Model file for the job. Use its own axes, mm. Face numbers are marked on the shaded views. Give positions to 0.01 mm unless a question says otherwise; leave off trailing zeros. Loops run counter-clockwise (first coordinate to the right, second up) from the corner with the lowest first, then second, coordinate; pieces in that order, holes last. Notation, with made-up numbers: (52.5, 34.25) -> (81.5, 34.25) arc R13 cw to (81.5, 50.25) -> close; hole circle Ø7 at (57.5, 77). An arc over 180 degrees is marked (long way). Use CSV: the item, a comma, the result in double quotes. Start each with the question number.
(1) Flat gauge pins, fed straight in: pin 1 (4.5 mm diameter, centred on y = -69.5, z = -6, fed in from -X); pin 2 (6 mm diameter, centred on x = 3.5, z = 4, fed in from +Y); pin 3 (3 mm diameter, centred on y = -69.5, z = -8.5, fed in from +X). Where does each tip first touch, or does it go through?
(2) Cut at A-A on y = 8. Write the cut outline in (x, z), then the cut area to 3 significant figures.
(3) Cut at B-B on z = -11.75. Write the cut outline in (x, y), then the cut area to 3 significant figures.
(4) Pull direction X, two halves, no side cores. Call the marked faces 1, 2, 3 and 4: pulls with the +X half, pulls with the -X half, needs draft (parallel to the pull), parting line crosses it, or undercut.
(5) Cut at C-C on x = 15. Write the cut outline in (y, z), then the cut area to 3 significant figures.
(6) Drill centre lines: probe 1 along Y at (x, z) = (1.5, -4.75); probe 2 along Y at (x, z) = (0, 8); probe 3 along Z at (x, y) = (-31, 64). Where is each one in solid material? Low to high.
(7) Cut at D-D on x = -64.5. Write the cut outline in (y, z), then the cut area to 3 significant figures.
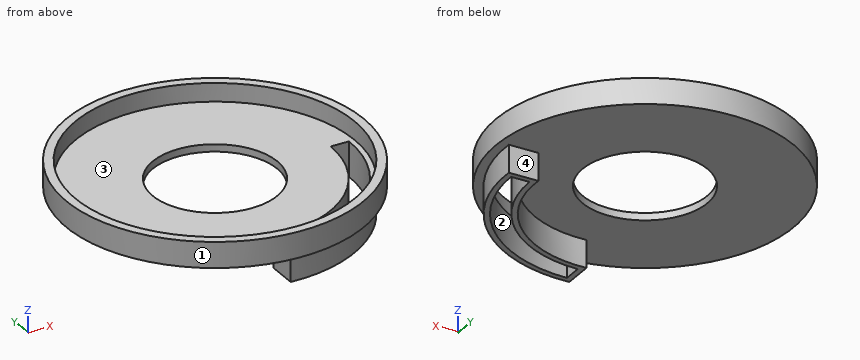
from build123d import *

# Parameters (mm, degrees)
SKETCH_1_R           = 76.1
SKETCH_1_R_2         = 34
EXTRUDE_1_DEPTH      = 4
EXTRUDE_2_DEPTH      = 10
EXTRUDE_2_DEPTH_BACK = 4
SKETCH_2_R           = 81.1
SKETCH_2_R_2         = 76.1
CUT_EXTRUDE_1_DEPTH  = 5
EXTRUDE_3_DEPTH      = 15


with BuildPart() as part:
    # 스케치1 → 보스-돌출1 (new body)
    with BuildSketch(Plane.XY):
        Circle(SKETCH_1_R)
        Circle(SKETCH_1_R_2, mode=Mode.SUBTRACT)
    extrude(amount=EXTRUDE_1_DEPTH)

    # 스케치2 → 보스-돌출2 (add, two sides: drawn at the far end of the back side and taken through both)
    with BuildSketch(Plane.XY.offset(4).offset(-EXTRUDE_2_DEPTH_BACK)):
        Circle(SKETCH_2_R)
        Circle(SKETCH_2_R_2, mode=Mode.SUBTRACT)
    extrude(amount=EXTRUDE_2_DEPTH + EXTRUDE_2_DEPTH_BACK)

    # 스케치3 → 컷-돌출1 (cut)
    with BuildSketch(Plane.XY.offset(4)):
        with BuildLine():
            Line((63, 0), (73.1, 0))
            ThreePointArc((73.1, 0), (51.689505705, -51.689505705), (0, -73.1))
            Line((0, -73.1), (0, -63))
            ThreePointArc((0, -63), (44.547727215, -44.547727215), (63, 0))
        make_face()
    extrude(amount=-CUT_EXTRUDE_1_DEPTH, mode=Mode.SUBTRACT)

    # 스케치4 → 보스-돌출3 (add)
    with BuildSketch(Plane(origin=(0, 0, 0), x_dir=(-1, 0, 0), z_dir=(0, 0, -1))):
        with BuildLine():
            Line((-59.924953066, 3), (-76.040844288, 3))
            ThreePointArc((-76.040844288, 3), (-53.810826048, -53.810826048), (3, -76.040844288))
            Line((3, -76.040844288), (3, -59.924953066))
            ThreePointArc((3, -59.924953066), (-42.426406871, -42.426406871), (-59.924953066, 3))
        make_face()
        with BuildLine():
            Line((-63, 0), (-73.1, 0))
            ThreePointArc((-73.1, 0), (-51.689505705, -51.689505705), (0, -73.1))
            Line((0, -73.1), (0, -63))
            ThreePointArc((0, -63), (-44.547727215, -44.547727215), (-63, 0))
        make_face(mode=Mode.SUBTRACT)
    extrude(amount=EXTRUDE_3_DEPTH)


solid = part.part
Check result:
1,pin 1,"x = -3"
1,pin 2,"y = 81.1"
1,pin 3,"x = 34.16"
2,outline,"(-80.7, 0) -> (-33.05, 0) -> (-33.05, 4) -> (-75.68, 4) -> (-75.68, 14) -> (-80.7, 14) -> close; (33.05, 0) -> (80.7, 0) -> (80.7, 14) -> (75.68, 14) -> (75.68, 4) -> (33.05, 4) -> close"
2,area,"482 mm²"
3,outline,"(-3, -76.04) arc R76.1 ccw to (76.04, 3) -> (59.92, 3) arc R60 cw to (-3, -59.92) -> close; hole (0, -73.1) arc R73.1 ccw to (73.1, 0) -> (63, 0) arc R63 cw to (0, -63) -> close"
3,area,"738 mm²"
4,face 1,"parting line crosses it"
4,face 2,"undercut"
4,face 3,"undercut"
4,face 4,"needs draft"
5,outline,"(-79.7, 0) -> (-74.61, 0) -> (-74.61, -15) -> (-71.54, -15) -> (-71.54, 4) -> (-74.61, 4) -> (-74.61, 14) -> (-79.7, 14) -> close; (-61.19, -15) -> (-58.09, -15) -> (-58.09, 0) -> (-30.51, 0) -> (-30.51, 4) -> (-61.19, 4) -> close; (30.51, 0) -> (79.7, 0) -> (79.7, 14) -> (74.61, 14) -> (74.61, 4) -> (30.51, 4) -> close"
5,area,"546 mm²"
6,probe 1,"-76.09 to -73.08, -62.98 to -59.98"
6,probe 2,"-81.1 to -76.1, 76.1 to 81.1"
6,probe 3,"0 to 4"
7,outline,"(-49.16, 0) -> (49.16, 0) -> (49.16, 14) -> (40.39, 14) -> (40.39, 4) -> (-40.39, 4) -> (-40.39, 14) -> (-49.16, 14) -> close"
7,area,"569 mm²"
